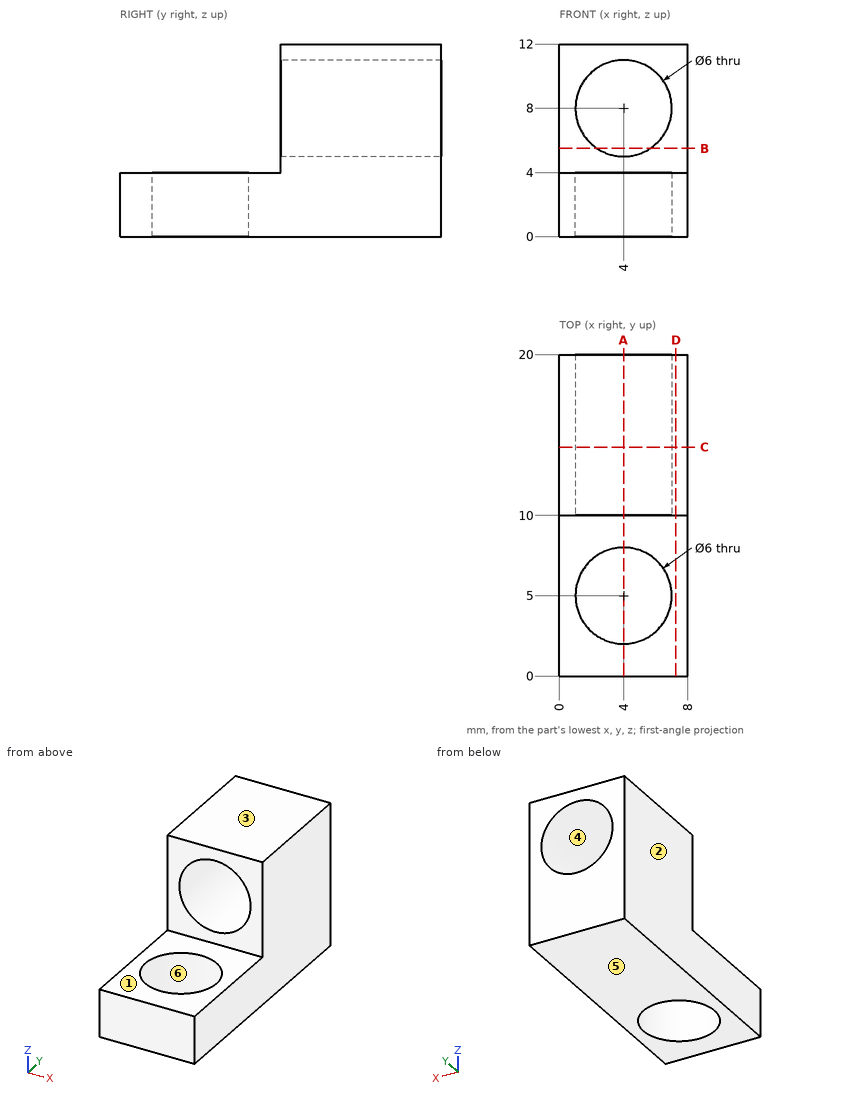
Source: three-view drawing plus pictorial views. Frame: mm from the lowest corner of the part. A direction names the side the tool comes from. Coordinates: 2 decimals unless noted, no trailing zeros. Loops run counter-clockwise (first coordinate to the right, second up) from the corner with the lowest first, then second, coordinate; pieces in that order, holes last. Notation, with made-up numbers: (-32.5, -6.75) - (6.5, -6.75) arc R18 ccw to (6.5, 2.25) - close; hole circle Ø6 at (26, -15). An arc over 180 degrees is marked (long way). One line per item, written item: value. Start each with the question number.
1. Ray query, L1, parallel to X at y = 13, z = 8; L2, parallel to Z at x = 1.5, y = 2.75; L3, parallel to Y at x = 5, z = 0.5. Return the intervals inside material, ascending.
2. Section D-D (x = 7.25). Return the cut outline in (y, z).
3. Set-up query: the marked faces 1 and 2. Return all of +Z, -Z, +X, -X, +Y, -Y with unobstructed straight access to the full face (end or side cutting, diameter ignored); none if empty.
4. Section A-A (x = 4). Return the cut outline in (y, z), and give its area (3 significant figures).
5. Section C-C (y = 14.25). Return the cut outline in (x, z), and give its area (3 significant figures).
6. Contact query for a flat-ended pin moving along its axis: P1, Ø1, axis at x = 5, z = 5.5, coming from the -Y side. Output: stop coordinate, or through.
7. Mould query, pull axis Z, two halves, no side actions, for the marked faces 3, 4, 5 and 6. Classes: pulls with the +Z half, pulls with the -Z half, needs draft (parallel to the pull), parting line crosses it, or undercut.
8. Section B-B (z = 5.5). Return the cut outline in (x, y), and give its area (3 significant figures).
Verdict:
1. L1: x = 0 to 1, 7 to 8
1. L2: z = 0 to 4
1. L3: y = 0 to 2.17, 7.83 to 20
2. outline: (0, 0) - (20, 0) - (20, 12) - (10, 12) - (10, 4) - (0, 4) - close
3. face 1: +Z, +X, -X, -Y
3. face 2: +Z, -Z, -X, +Y, -Y
4. outline: (0, 0) - (2, 0) - (2, 4) - (0, 4) - close; (8, 0) - (20, 0) - (20, 5) - (10, 5) - (10, 4) - (8, 4) - close; (10, 11) - (20, 11) - (20, 12) - (10, 12) - close
4. area: 76.0 mm2
5. outline: (0, 0) - (8, 0) - (8, 12) - (0, 12) - close; hole circle Ø6 at (4, 8)
5. area: 67.7 mm2
6. P1: stops at y = 10
7. face 3: pulls with the +Z half
7. face 4: undercut
7. face 5: pulls with the -Z half
7. face 6: needs draft
8. outline: (0, 10) - (2.34, 10) - (2.34, 20) - (0, 20) - close; (5.66, 10) - (8, 10) - (8, 20) - (5.66, 20) - close
8. area: 46.8 mm2
